```python
from build123d import *

# Parameters (mm, degrees)
BOX_W        = 51
BOX_H        = 10.2
BOX_DEPTH    = 10
BOX001_W     = 51
BOX001_H     = 13.2
BOX001_DEPTH = 10
BOX002_W     = 57
BOX002_H     = 33
BOX002_DEPTH = 6


with BuildPart() as cube:
    # Box → Box (new body)
    with BuildSketch(Plane.XY.offset(-7)):
        with Locations((25.5, 5.1)):
            Rectangle(BOX_W, BOX_H)
    extrude(amount=BOX_DEPTH)


with BuildPart() as fusion:
    # Box001 → Box001 (new body)
    with BuildSketch(Plane(origin=(0, -17.2, -7), x_dir=(1, 0, 0), z_dir=(0, 0, 1))):
        with Locations((25.5, 6.6)):
            Rectangle(BOX001_W, BOX001_H)
    extrude(amount=BOX001_DEPTH)

    # Fusion: union Cube
    add(cube.part)


with BuildPart() as cut:
    # Box002 → Box002 (new body)
    with BuildSketch(Plane(origin=(-3, -20, 0), x_dir=(1, 0, 0), z_dir=(0, 0, 1))):
        with Locations((28.5, 16.5)):
            Rectangle(BOX002_W, BOX002_H)
    extrude(amount=BOX002_DEPTH)

    # Cut: cut Fusion
    add(fusion.part, mode=Mode.SUBTRACT)


solid = cut.part
```
Geometry check sheet. Reference: the model listing, model coordinates, mm. A direction names the side the tool comes from. Give positions to 0.01 mm unless a question says otherwise; leave off trailing zeros. Write each loop counter-clockwise with the first axis right and the second up, starting at its lowest first coordinate (ties: lowest second). Pieces come first, ordered by that corner, then holes.
1) Section check B-B, the plane x = 48. Record the boundary of the cut face in (y, z), and give its area (3 significant figures).
2) Section check C-C, the plane y = -16.5. Record the boundary of the cut face in (x, z), and give its area (3 significant figures).
3) Section check A-A, the plane z = 0.8. Record the boundary of the cut face in (x, y), and give its area (3 significant figures).
4) Release check for a two-part mould opening along Y. For faces 1 (the flat face through (25, 10.2, 1)), 2 (the flat face through (25, 0, 1)), 3 (the flat face through (54, -4, 3)), 4 (the flat face through (25, -20, 3)) record: pulls with the +Y half, pulls with the -Y half, needs draft (parallel to the pull), parting line crosses it, or undercut.
5) Access from +Z, -Z, +X, -X, +Y, -Y to the whole of each face (thin tool, end or side, straight path). Record for faces 5 (the flat face through (51, 5, 1)), 6 (the flat face through (25, 13, 3)).
6) Gauge pin test, flat end, axial feed: pin 1 (1.5 mm diameter, centred on x = 21.5, y = -8.5, fed in from -Z). Record the tip position at first contact, or that the pin passes through.
7) Material ranges on L1, parallel to Y at x = 17, z = 0.8; L2, parallel to X at y = -7.5, z = 1.8; L3, parallel to Z at x = 9.5, y = -16, recorded low to high.
Computed:
1. outline: (-20, 0) - (-17.2, 0) - (-17.2, 3) - (-4, 3) - (-4, 0) - (0, 0) - (0, 3) - (10.2, 3) - (10.2, 0) - (13, 0) - (13, 6) - (-20, 6) - close
1. area: 128 mm2
2. outline: (-3, 0) - (0, 0) - (0, 3) - (51, 3) - (51, 0) - (54, 0) - (54, 6) - (-3, 6) - close
2. area: 189 mm2
3. outline: (-3, -20) - (54, -20) - (54, 13) - (-3, 13) - close; hole (0, -17.2) - (51, -17.2) - (51, -4) - (0, -4) - close; hole (0, 0) - (51, 0) - (51, 10.2) - (0, 10.2) - close
3. area: 688 mm2
4. face 1: undercut
4. face 2: undercut
4. face 3: needs draft
4. face 4: pulls with the -Y half
5. face 5: -Z
5. face 6: +Z, -Z, +X, -X, +Y
6. pin 1: stops at z = 3
7. L1: y = -20 to -17.2, -4 to 0, 10.2 to 13
7. L2: x = -3 to 0, 51 to 54
7. L3: z = 3 to 6
